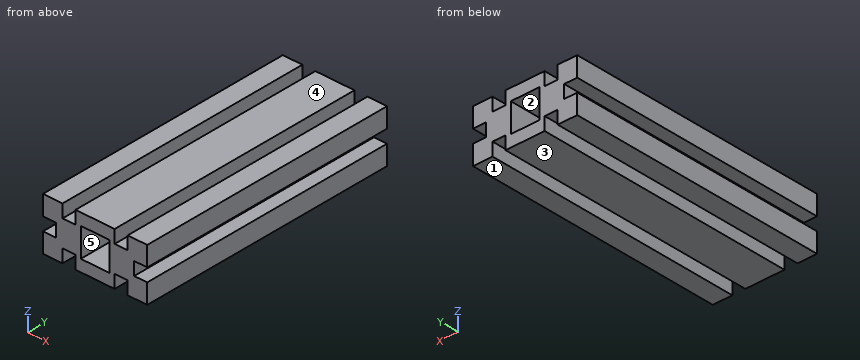
```python
from build123d import *

# Parameters (mm, degrees)
SKETCH1_W       = 40
SKETCH1_H       = 20
BODY_DEPTH      = 100
SKETCH2_W       = 5
SKETCH2_H       = 5
SKETCH2_W_2     = 11
SKETCH2_H_2     = 11
PROFILAGE_DEPTH = 103.46950766


with BuildPart() as part:
    # Sketch1 → Body (new body)
    with BuildSketch(Plane(origin=(0, 0, 0), x_dir=(1, 0, 0), z_dir=(0, 1, 0))):
        Rectangle(SKETCH1_W, SKETCH1_H)
    extrude(amount=BODY_DEPTH)

    # Sketch2 → Profilage (cut, through all)
    with BuildSketch(Plane(origin=(0, 100, 0), x_dir=(1, 0, 0), z_dir=(0, 1, 0))):
        with Locations((-10, 7.5)):
            Rectangle(SKETCH2_W, SKETCH2_H)
        with Locations((-17.5, 0)):
            Rectangle(SKETCH2_W, SKETCH2_H)
        with Locations((-10, -7.5)):
            Rectangle(SKETCH2_W, SKETCH2_H)
        with Locations((10, -7.5)):
            Rectangle(SKETCH2_W, SKETCH2_H)
        with Locations((17.5, 0)):
            Rectangle(SKETCH2_W, SKETCH2_H)
        with Locations((10, 7.5)):
            Rectangle(SKETCH2_W, SKETCH2_H)
        Rectangle(SKETCH2_W_2, SKETCH2_H_2)
    extrude(amount=-PROFILAGE_DEPTH, mode=Mode.SUBTRACT)


solid = part.part
```
Check sheet for the modelled part. Datum: model origin and axes. Units: mm. Face numbers are marked on the shaded views. A direction names the side the tool comes from. Coordinates: 2 decimals unless noted, no trailing zeros. Write each loop counter-clockwise with the first axis right and the second up, starting at its lowest first coordinate (ties: lowest second). Pieces come first, ordered by that corner, then holes. Notation, with made-up numbers: M 0.25,-21 L 29.25,-21 A22 cw 29.25,-4 Z; hole C 35,79 d5. An arc over 180 degrees is marked long. Use one line per item in the form item = value.
Item 1: Gauge pin test, flat ends, axial feed: pin 1 Ø1.5 at (y, z) = (33.5, 1) entering from +X; pin 2 Ø1.5 at (x, z) = (-0.5, 6.5) entering from -Y; pin 3 Ø1.5 at (x, z) = (3, 0) entering from +Y; pin 4 Ø2.5 at (x, y) = (-9, 56) entering from +Z. Record the tip position at first contact, or that the pin passes through.
Answer below:
pin_1 = 15
pin_2 = 0
pin_3 = through
pin_4 = 5
Item 2: Set-up check for the marked faces 1 and 2: record each of +Z, -Z, +X, -X, +Y, -Y from which the full face is reachable in a straight line by a thin tool's end or side.
Answer below:
face_1 = -Z, +X, -X, +Y, -Y
face_2 = +Y, -Y
Item 3: Material ranges on L1, parallel to X at y = 75, z = 7.5; L2, parallel to Z at x = 2.5, y = 41.5; L3, parallel to X at y = 57, z = -4.25, recorded low to high. Write a range as from..to.
Answer below:
L1 = -20..-12.5, -7.5..7.5, 12.5..20
L2 = -10..-5.5, 5.5..10
L3 = -20..-5.5, 5.5..20
Item 4: Sectioned sample at A-A, the plane z = 8.25. Record the cut outline in (x, y), and give its area (3 significant figures).
Answer below:
outline = M -20,0 L -12.5,0 L -12.5,100 L -20,100 Z; M -7.5,0 L 7.5,0 L 7.5,100 L -7.5,100 Z; M 12.5,0 L 20,0 L 20,100 L 12.5,100 Z
area = 3,000 mm^2
Item 5: Release check for a two-part mould opening along Z. For the marked faces 3, 4 and 5 record: pulls with the +Z half, pulls with the -Z half, needs draft (parallel to the pull), parting line crosses it, or undercut.
Answer below:
face_3 = pulls with the -Z half
face_4 = pulls with the +Z half
face_5 = undercut
Item 6: Sectioned sample at C-C, the plane x = 4. Record the cut outline in (y, z).
Answer below:
outline = M 0,-10 L 100,-10 L 100,-5.5 L 0,-5.5 Z; M 0,5.5 L 100,5.5 L 100,10 L 0,10 Z
